Source: three-view drawing plus pictorial views. Frame: mm from the lowest corner of the part. Coordinates: 2 decimals unless noted, no trailing zeros. Loops run counter-clockwise (first coordinate to the right, second up) from the corner with the lowest first, then second, coordinate; pieces in that order, holes last. Notation, with made-up numbers: M -17.5,80.25 L 36.5,80.25 A26 cw 36.5,119.25 Z; hole C 4.25,79.5 d11. An arc over 180 degrees is marked long. Use a Markdown table: item, result. Add a question column.
1. Line query: L1, parallel to Z at x = 250, y = 15.25; L2, parallel to X at y = 4, z = 260; L3, parallel to X at y = 12, z = 137. Output: solid intervals per line, ascending. Write a range as [from, to].
2. Section B-B on z = 140. Output: boundary loops of the cut face in (x, y).
3. Section A-A on x = 250. Output: boundary loops of the cut face in (y, z).
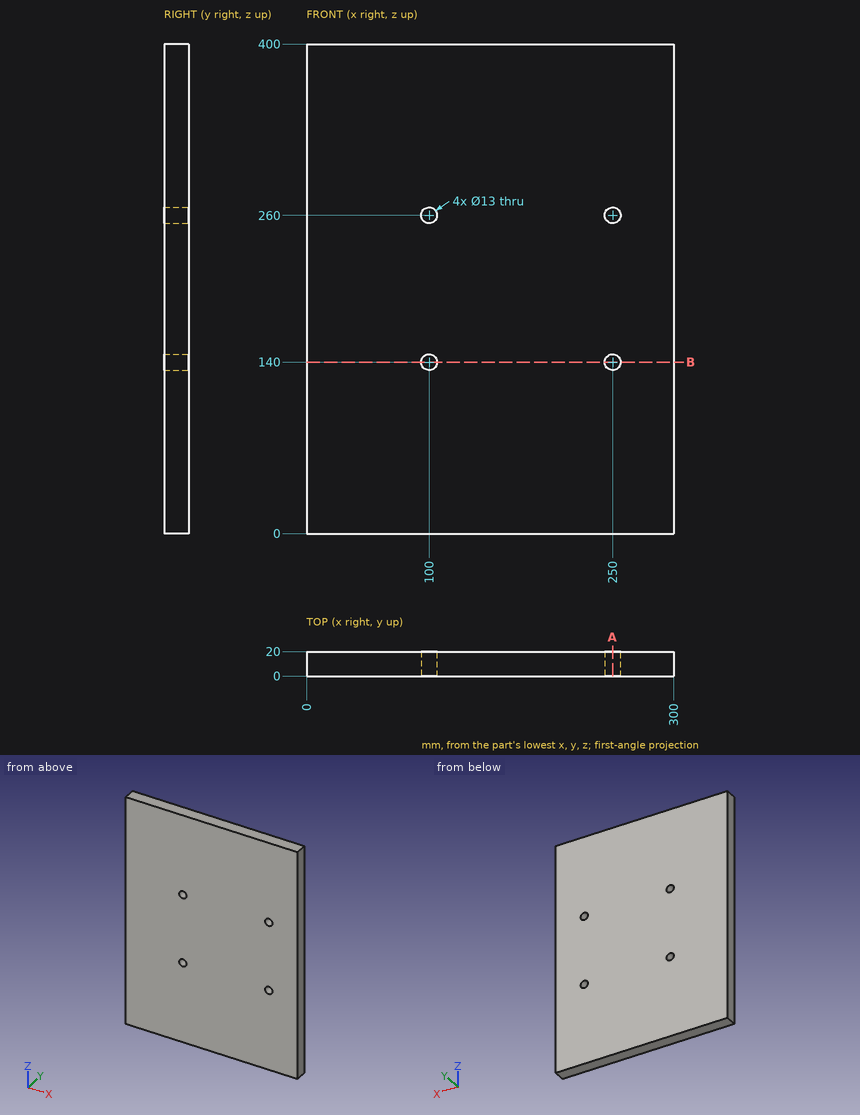
Answers below:
| question | item | result |
|---|---|---|
| 1 | L1 | z = [0, 133.5], [146.5, 253.5], [266.5, 400] |
| 1 | L2 | x = [0, 93.5], [106.5, 243.5], [256.5, 300] |
| 1 | L3 | x = [0, 94.23], [105.77, 244.23], [255.77, 300] |
| 2 | outline | M 0,0 L 93.5,0 L 93.5,20 L 0,20 Z; M 106.5,0 L 243.5,0 L 243.5,20 L 106.5,20 Z; M 256.5,0 L 300,0 L 300,20 L 256.5,20 Z |
| 3 | outline | M 0,0 L 20,0 L 20,133.5 L 0,133.5 Z; M 0,146.5 L 20,146.5 L 20,253.5 L 0,253.5 Z; M 0,266.5 L 20,266.5 L 20,400 L 0,400 Z |
